Solid Edge part; units mm, degrees
sketch "Sketch1" plane through (0, 0, 0) normal (0, 0, 1) x (1, 0, 0)
  line L0 (10, -10) -> (-10, -10)
  line L1 (-10, -10) -> (-10, 10)
  line L2 (-10, 10) -> (10, 10)
  line L3 (10, 10) -> (10, -10)
extrude "Protrusion1" add sketch "Sketch1" against normal blind 3
sketch "Sketch2" plane through (0, 0, 0) normal (0, 0, 1) x (1, 0, 0)
  line L0 (8, -8) -> (-8, -8)
  line L1 (-8, -8) -> (-8, 8)
  line L2 (-8, 8) -> (8, 8)
  line L3 (8, 8) -> (8, -8)
  circle A0 centre (0, 0) radius 7
extrude "ExtrudedProtrusion_2" add sketch "Sketch2" along normal blind 15
fillet "Round_1" radius 2 8 edges at (10, -10, -1.5) (10, 10, -1.5) (-10, -10, -1.5) (-10, 10, -1.5) (-8, 8, 7.5) (-8, -8, 7.5) (8, -8, 7.5) (8, 8, 7.5)
fillet "Round_2" radius 1 8 edges at (-10, 0, -3) (-9.4142, 9.4142, -3) (0, 10, -3) (9.4142, 9.4142, -3) (10, 0, -3) (9.4142, -9.4142, -3) (0, -10, -3) (-9.4142, -9.4142, -3)
Geometry: final body of the model. Coordinates: model frame, mm. A direction names the side the tool comes from. Round coordinates to 2 decimals unless told otherwise and drop trailing zeros. Loops run counter-clockwise (first coordinate to the right, second up) from the corner with the lowest first, then second, coordinate; pieces in that order, holes last. Notation, with made-up numbers: (1.5, 43) -> (46.5, 43) arc R34 ccw to (46.5, 76) -> close; hole circle Ø3 at (47.25, 55). An arc over 180 degrees is marked (long way). Write each question's results on one line, items separated by ' | '.
Item 1: Set-up query: faces 5 (the face through (7.43, 7.4, 7.6)), 6 (the face through (0, -8, 7)), 7 (the face through (-7.4, 7.43, 7.6)), 8 (the face through (-7.43, -7.4, 7.6)), 9 (the face through (8, 0, 7)). Return all of +Z, -Z, +X, -X, +Y, -Y with unobstructed straight access to the full face (end or side cutting, diameter ignored); none if empty.
Answers below:
face 5: +Z, +X, +Y | face 6: +Z, +X, -X, -Y | face 7: +Z, -X, +Y | face 8: +Z, -X, -Y | face 9: +Z, +X, +Y, -Y
Item 2: Cut plane B-B on y = 0. Return the cut outline in (x, z), and give its area (3 significant figures).
Answers below:
outline: (-10, -2) arc R1 ccw to (-9, -3) -> (9, -3) arc R1 ccw to (10, -2) -> (10, 0) -> (8, 0) -> (8, 15) -> (7, 15) -> (7, 0) -> (-7, 0) -> (-7, 15) -> (-8, 15) -> (-8, 0) -> (-10, 0) -> close | area: 89.6 mm²
Item 3: Line query: probe 1 along Y at (x, z) = (0, 8.5); probe 2 along Z at (x, y) = (5.5, 1); probe 3 along X at (y, z) = (1.5, 13). Output: solid intervals per line, ascending. Write a range as [from, to].
Answers below:
probe 1: y = [-8, -7], [7, 8] | probe 2: z = [-3, 0] | probe 3: x = [-8, -6.84], [6.84, 8]
Item 4: Cut plane A-A on z = 5.75. Return the cut outline in (x, y).
Answers below:
outline: (-8, -6) arc R2 ccw to (-6, -8) -> (6, -8) arc R2 ccw to (8, -6) -> (8, 6) arc R2 ccw to (6, 8) -> (-6, 8) arc R2 ccw to (-8, 6) -> close; hole circle Ø14 at (0, 0)
Item 5: Pin query (flat end, axial travel): pin 1 Ø6 at (x, z) = (-3.5, 10.5) entering from +Y; pin 2 Ø6 at (y, z) = (2, 9.5) entering from +X; pin 3 Ø3.5 at (y, z) = (2, 4.5) entering from -X. Return the tip coordinate at first contact, or that it passes through.
Answers below:
pin 1: stops at y = 8 | pin 2: stops at x = 8 | pin 3: stops at x = -8
Item 6: Pull-direction query (Y, two-part tool) for faces 1 (the face through (0, 0, -3)), 2 (the face through (0, 0, 0)), 3 (the face through (6.466, 2.681, 7.395)), 4 (the face through (0.112, 9.699, -2.715)); classes: pulls with the +Y half, pulls with the -Y half, needs draft (parallel to the pull), parting line crosses it, or undercut.
Answers below:
face 1: needs draft | face 2: undercut | face 3: undercut | face 4: pulls with the +Y half
